Verification items for the finished model (mm, model axes). Round coordinates to 2 decimals unless told otherwise and drop trailing zeros. Write each loop counter-clockwise with the first axis right and the second up, starting at its lowest first coordinate (ties: lowest second). Pieces come first, ordered by that corner, then holes. Notation, with made-up numbers: (-10, 63) -> (28, 63) arc R23 ccw to (28, 78) -> close; hole circle Ø11 at (59.5, -33.75). An arc over 180 degrees is marked (long way). Answer as a JSON object with one key per item and string values. Group by question number.
(1) Sectioned sample at A-A on x = -46.5. Record the cut outline in (y, z).
(2) Scan lines: L1, parallel to X at y = 3.5, z = -77.5; L2, parallel to X at y = 2.25, z = -75. Record each from-to range of solid material in increasing order. Write a range as from..to.
(3) Gauge pin test, flat ends, axial feed: pin 1 Ø1.8 at (x, y) = (-114.89, 6) entering from +Z; pin 2 Ø3.5 at (x, y) = (-35.5, 5.5) entering from +Z; pin 3 Ø0.9 at (y, z) = (6, -192.5) entering from +X. Record the tip position at first contact, or that the pin passes through.
```python
from build123d import *

# Parameters (mm, degrees)
SKETCH1_W           = 134
SKETCH1_H           = 168
SKETCH1_R           = 7
BOSS_EXTRUDE1_DEPTH = 12
CUT_EXTRUDE1_START  = -44.256673
SKETCH2_R           = 1.5
CUT_EXTRUDE1_DEPTH  = 20
CUT_EXTRUDE2_START  = -20.894163
SKETCH3_R           = 1.5
CUT_EXTRUDE2_DEPTH  = 20


with BuildPart() as part:
    # Sketch1 → Boss-Extrude1 (new body)
    with BuildSketch(Plane(origin=(0, 0, 0), x_dir=(1, 0, 0), z_dir=(0, 1, 0))):
        with Locations((-87.894163325, 128.256672781)):
            Rectangle(SKETCH1_W, SKETCH1_H)
        with Locations((-47.894163325, 71.256672781)):
            Circle(SKETCH1_R, mode=Mode.SUBTRACT)
    extrude(amount=BOSS_EXTRUDE1_DEPTH)

    # Sketch2 → Cut-Extrude1 (cut)
    with BuildSketch(Plane.XY.offset(CUT_EXTRUDE1_START)):
        with Locations((-114.894163325, 6)):
            Circle(SKETCH2_R)
        with Locations((-35.894163325, 6)):
            Circle(SKETCH2_R)
    extrude(amount=-CUT_EXTRUDE1_DEPTH, mode=Mode.SUBTRACT)

    # Sketch3 → Cut-Extrude2 (cut)
    with BuildSketch(Plane(origin=(0, 0, 0), x_dir=(0, 0, -1), z_dir=(1, 0, 0)).offset(CUT_EXTRUDE2_START)):
        with Locations((192.256672781, 6)):
            Circle(SKETCH3_R)
    extrude(amount=-CUT_EXTRUDE2_DEPTH, mode=Mode.SUBTRACT)


solid = part.part
```
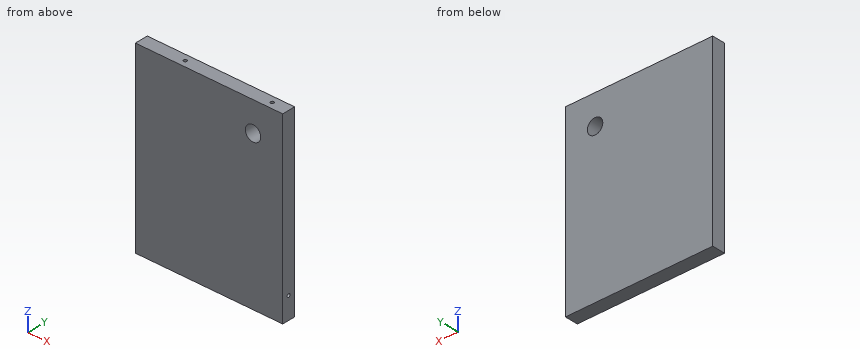
Computed values:
{
 "1": {"outline": "(0, -212.26) -> (12, -212.26) -> (12, -78.12) -> (0, -78.12) -> close; (0, -64.4) -> (12, -64.4) -> (12, -44.26) -> (0, -44.26) -> close"},
 "2": {"L1": "-154.89..-51.06, -44.73..-20.89", "L2": "-154.89..-53.81, -41.98..-20.89"},
 "3": {"pin 1": "z = -64.26", "pin 2": "z = -44.26", "pin 3": "x = -40.89"}
}
